from build123d import *

# Parameters (mm, degrees)
F1_DEPTH       = 4
F2_D           = 5.5
F2_CSINK_D     = 11.2
F2_CSINK_ANGLE = 90


with BuildPart() as f1:
    # F0 (on Front) → F1 (new body)
    with BuildSketch(Plane.XZ):
        Polygon((15, 0), (15, 17.5), (-15, 17.5), (-15, 0), (-55, 0), (-55, -17.5), (55, -17.5), (55, 0), align=None)
    extrude(amount=F1_DEPTH)

    # F2 (through all)
    with Locations(Plane(origin=(0, 0, 0), x_dir=(1, 0, 0), z_dir=(0, 1, 0))):
        with Locations((0, -10.25), (0, 10.25)):
            CounterSinkHole(F2_D / 2, F2_CSINK_D / 2, counter_sink_angle=F2_CSINK_ANGLE)


solid = f1.part
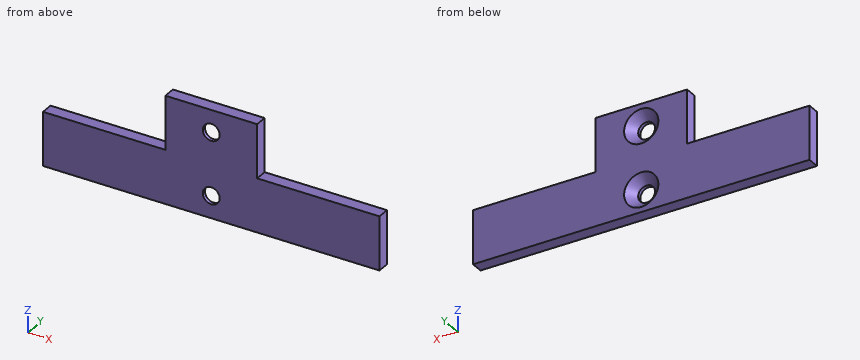
Geometry: final body of the model. Coordinates: model frame, mm. Coordinates: 2 decimals unless noted, no trailing zeros. Loops run counter-clockwise (first coordinate to the right, second up) from the corner with the lowest first, then second, coordinate; pieces in that order, holes last. Notation, with made-up numbers: (50.5, -25) - (61.5, -25) arc R10 ccw to (61.5, -21) - close; hole circle Ø11 at (-21.5, 29). An arc over 180 degrees is marked (long way). Put each result on its own line as item: value. Start each with the question number.
Q1. Cut plane B-B, the plane x = 0. Return loops of the section in (y, z), and give its area (3 significant figures).
Q2. Cut plane A-A, the plane z = -10.25. Return loops of the section in (x, y).
Q3. Cut plane D-D, the plane z = 10.25. Return loops of the section in (x, y), and give its area (3 significant figures).
Q4. Cut plane C-C, the plane y = -1.7. Return loops of the section in (x, z).
Q5. Line query: line 1 (Z direction, x = 0, y = -3.2); line 2 (X direction, y = -3.7, z = 10.25); line 3 (X direction, y = -1.4, z = -12). Output: solid intervals per line, ascending.
Q6. Pin query (flat end, axial travel): pin 1 Ø1.2 at (x, y) = (-36.5, -3) entering from +Z; pin 2 Ø1.2 at (y, z) = (-2, 9) entering from +X; pin 3 Ø1.5 at (x, z) = (-20.5, 0) entering from +Y; pin 4 Ø9 at (x, z) = (0, 10.25) entering from +Y. Return the tip coordinate at first contact, or that it passes through.
Filled sheet:
1. outline: (-4, -17.5) - (0, -17.5) - (0, -15.85) - (-2.85, -13) - (-4, -13) - close; (-4, -7.5) - (-2.85, -7.5) - (0, -4.65) - (0, 4.65) - (-2.85, 7.5) - (-4, 7.5) - close; (-4, 13) - (-2.85, 13) - (0, 15.85) - (0, 17.5) - (-4, 17.5) - close
1. area: 79.8 mm²
2. outline: (-55, -4) - (-2.75, -4) - (-2.75, -2.85) - (-5.6, 0) - (-55, 0) - close; (2.75, -4) - (55, -4) - (55, 0) - (5.6, 0) - (2.75, -2.85) - close
3. outline: (-15, -4) - (-2.75, -4) - (-2.75, -2.85) - (-5.6, 0) - (-15, 0) - close; (2.75, -4) - (15, -4) - (15, 0) - (5.6, 0) - (2.75, -2.85) - close
3. area: 89.9 mm²
4. outline: (-55, -17.5) - (55, -17.5) - (55, 0) - (15, 0) - (15, 17.5) - (-15, 17.5) - (-15, 0) - (-55, 0) - close; hole circle Ø7.8 at (0, -10.25); hole circle Ø7.8 at (0, 10.25)
5. line 1: -17.5 to -13, -7.5 to 7.5, 13 to 17.5
5. line 2: -15 to -2.75, 2.75 to 15
5. line 3: -55 to -3.82, 3.82 to 55
6. pin 1: z = 0
6. pin 2: x = 15
6. pin 3: y = 0
6. pin 4: y = -1.1
